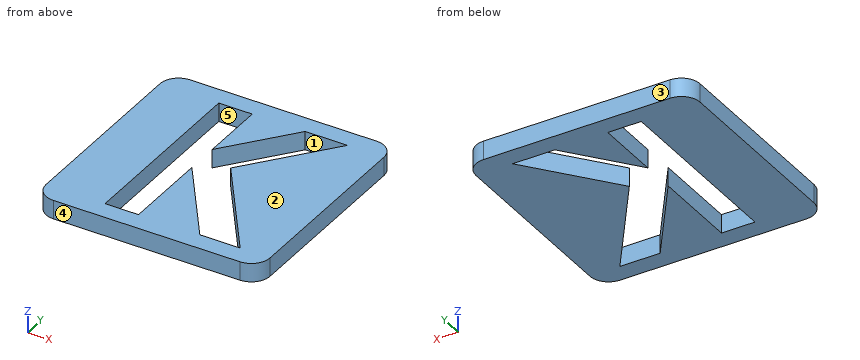
```python
from build123d import *

# Parameters (mm, degrees)
BOSS_EXTRUDE1_DEPTH = 10
CUT_EXTRUDE24_DEPTH = 10


with BuildPart() as part:
    # Sketch1 → Boss-Extrude1 (new body)
    with BuildSketch(Plane.XY):
        with BuildLine():
            Line((-50, 60), (50, 60))
            ThreePointArc((50, 60), (57.071067812, 57.071067812), (60, 50))
            Line((60, 50), (60, -50))
            ThreePointArc((60, -50), (57.071067812, -57.071067812), (50, -60))
            Line((50, -60), (-50, -60))
            ThreePointArc((-50, -60), (-57.071067812, -57.071067812), (-60, -50))
            Line((-60, -50), (-60, 50))
            ThreePointArc((-60, 50), (-57.071067812, 57.071067812), (-50, 60))
        make_face()
    extrude(amount=BOSS_EXTRUDE1_DEPTH)

    # Sketch2 → Cut-Extrude24 (cut)
    with BuildSketch(Plane.XY.offset(10)):
        Polygon((-28.461538462, 50), (-10.512820513, 50), (-10.512820513, 14.803685897), (17.852564103, 50), (40.508814103, 50), (4.871794872, 5.769230769), (43.974358974, -50), (22.359775641, -50), (-10.512820513, -3.104967949), (-10.512820513, -50), (-28.461538462, -50), align=None)
    extrude(amount=-CUT_EXTRUDE24_DEPTH, mode=Mode.SUBTRACT)


solid = part.part
```
Can you work these out from the model? Positions are in its coordinate system, mm. Face numbers are marked on the shaded views. A direction names the side the tool comes from. Round coordinates to 2 decimals unless told otherwise and drop trailing zeros. Loops run counter-clockwise (first coordinate to the right, second up) from the corner with the lowest first, then second, coordinate; pieces in that order, holes last. Notation, with made-up numbers: M -16.75,19 L 23.25,19 A10 ccw 23.25,26 Z; hole C 56.5,77 d6. An arc over 180 degrees is marked long. Answer as a JSON object with one key per item and string values. Group by question number.
Q1. On a 3-axis mill with a long thin cutter (end or side, diameter ignored), from which of +Z, -Z, +X, -X, +Y, -Y can I reach the whole of each face in a straight line? I mean the marked faces 1 and 2. Say none if no direction works.
Q2. Imagine slicing it at A-A, the plane x = -19. Please give me the cut outline in (y, z).
Q3. Imagine slicing it at D-D, the plane x = 7.5. Please give me the cut outline in (y, z), then the cut area to 3 significant figures.
Q4. Imagine slicing it at C-C, the plane y = 12. Please give me the cut outline in (x, z), then the cut area to 3 significant figures.
Q5. Please list where these lines run through material, in increasing order: L1, parallel to Y at x = -17, z = 4.75; L2, parallel to Y at x = 8, z = 1.75; L3, parallel to X at y = -27.5, z = 7.5.
Q6. We'd pull the mould along Y, two halves only. Please class the marked faces 3, 4 and 5: +Y half, -Y half, draft (parallel to the pull), parting line (faces both ways), or undercut.
Q7. Will this pin go through, and if not, where does the flat tip stop? pin 1 (2 mm diameter, centred on x = -0.5, y = -14.5, fed in from +Z).
Q8. Imagine slicing it at B-B, the plane z = 8.25. Please give me the cut outline in (x, y).
Findings:
{
 "1": {"face 1": "+Z, -Z", "face 2": "+Z, +X, -X, +Y, -Y"},
 "2": {"outline": "M -60,0 L -50,0 L -50,10 L -60,10 Z; M 50,0 L 60,0 L 60,10 L 50,10 Z"},
 "3": {"outline": "M -60,0 L -28.8,0 L -28.8,10 L -60,10 Z; M 2.02,0 L 9.03,0 L 9.03,10 L 2.02,10 Z; M 37.15,0 L 60,0 L 60,10 L 37.15,10 Z", "area": "611 mm2"},
 "4": {"outline": "M -60,0 L -28.46,0 L -28.46,10 L -60,10 Z; M 9.89,0 L 60,0 L 60,10 L 9.89,10 Z", "area": "816 mm2"},
 "5": {"L1": "y = -60 to -50, 50 to 60", "L2": "y = -60 to -29.51, 1.31 to 9.65, 37.77 to 60", "L3": "x = -60 to -28.46, -10.51 to 6.59, 28.2 to 60"},
 "6": {"face 3": "+Y half", "face 4": "-Y half", "face 5": "undercut"},
 "7": {"pin 1": "passes through"},
 "8": {"outline": "M -60,-50 A10 ccw -50,-60 L 50,-60 A10 ccw 60,-50 L 60,50 A10 ccw 50,60 L -50,60 A10 ccw -60,50 Z; hole M -28.46,-50 L -10.51,-50 L -10.51,-3.1 L 22.36,-50 L 43.97,-50 L 4.87,5.77 L 40.51,50 L 17.85,50 L -10.51,14.8 L -10.51,50 L -28.46,50 Z"}
}
